Check sheet for the modelled part. Datum: model origin and axes. Units: mm. A direction names the side the tool comes from. Round coordinates to 2 decimals unless told otherwise and drop trailing zeros. Order: outer loops, then holes, each group sorted by start corner. A loop starts at its lowest first (then second) coordinate and runs counter-clockwise, first axis right, second up. Notation, with made-up numbers: M 43.25,8.5 L 54.25,8.5 A6 cw 54.25,13.5 Z; hole C -17,0 d3. An arc over 180 degrees is marked long. One line per item, written item: value. Start each with the question number.
(1) Cross-section at B-B, the plane z = 0. Enter the section's corners in (x, y) (3 decimals), and give its area (3 significant figures).
(2) Cross-section at C-C, the plane y = 3.25. Enter the section's corners in (x, z), and give its area (3 significant figures).
(3) Access from +Z, -Z, +X, -X, +Y, -Y to the whole of each face (thin tool, end or side, straight path). Record for faces 4 (the face through (4, 8, -5)), 5 (the face through (0, 10, -9.975)).
(4) Cross-section at A-A, the plane x = 0. Enter the section's corners in (y, z) (3 decimals).
(5) Depth check by flat-ended pin: pin 1 Ø4 at (x, y) = (-5, 4) entering from -Z; pin 2 Ø3 at (x, y) = (-0.5, 7) entering from +Z (3 decimals); pin 3 Ø4 at (x, y) = (-3, 5.5) entering from -Z. Enter the tip coordinate at first touch or a pass-through.
(6) Thickness scan on L1, parallel to X at y = 5, z = 0; L2, parallel to Y at x = -1.5, z = 6.25; L3, parallel to X at y = 10.25, z = 2.75 (3 decimals). Record the ranges inside material, lowest first.
(7) Release check for a two-part mould opening along X. For faces 1 (the face through (-1.802, 4.056, -5.723)), 2 (the face through (0, 10.5, 0)), 3 (the face through (0, 10, 9.975)) record: released by +X, released by -X, zero draft, split by the parting line, or undercut.
(8) Cross-section at D-D, the plane x = -8.5. Enter the section's corners in (y, z) (3 decimals), and give its area (4 significant figures).
from build123d import *

# Parameters (mm, degrees)
CROQUIS1_W              = 6
CROQUIS1_H              = 8
CROQUIS2_W              = 19.95
CROQUIS2_H              = 19.95
SALIENTE_EXTRUIR1_DEPTH = 5
SKETCH6_R               = 4
CUT_EXTRUDE1_DEPTH      = 10.5


with BuildPart() as part:
    # Croquis1 → Revolución1 (revolve)
    with BuildSketch(Plane(origin=(0, 0, 0), x_dir=(0, 0, -1), z_dir=(1, 0, 0)), mode=Mode.PRIVATE) as revoluci_n1_sk:
        with Locations((-3, 4)):
            Rectangle(CROQUIS1_W, CROQUIS1_H)
    revolve(revoluci_n1_sk.sketch.rotate(Axis((0, 0, 0), (0, 1, 0)), 180), axis=Axis((0, 0, 0), (0, 1, 0)))

    # Croquis2 → Saliente-Extruir1 (add)
    with BuildSketch(Plane(origin=(0, 8, 0), x_dir=(1, 0, 0), z_dir=(0, 1, 0))):
        Rectangle(CROQUIS2_W, CROQUIS2_H)
    extrude(amount=SALIENTE_EXTRUIR1_DEPTH)

    # Sketch6 → Cut-Extrude1 (cut)
    with BuildSketch(Plane.XZ):
        with Locations(Location((0, 0, 0), (0, 0, 270))):
            Circle(SKETCH6_R)
    extrude(amount=-CUT_EXTRUDE1_DEPTH, mode=Mode.SUBTRACT)


solid = part.part
Values found:
1. outline: M -9.975,8 L -6,8 L -6,0 L -4,0 L -4,10.5 L 4,10.5 L 4,0 L 6,0 L 6,8 L 9.975,8 L 9.975,13 L -9.975,13 Z
1. area: 112 mm^2
2. outline: C 0,0 d12; hole C 0,0 d8
2. area: 62.8 mm^2
3. face 4: -Y
3. face 5: -Z, +X, -X, +Y, -Y
4. outline: M 0,-6 L 8,-6 L 8,-9.975 L 13,-9.975 L 13,9.975 L 8,9.975 L 8,6 L 0,6 L 0,4 L 10.5,4 L 10.5,-4 L 0,-4 Z
5. pin 1: z = -5.2
5. pin 2: z = 9.975
5. pin 3: z = -5.92
6. L1: -6 to -4, 4 to 6
6. L2: 8 to 13
6. L3: -9.975 to -2.905, 2.905 to 9.975
7. face 1: split by the parting line
7. face 2: undercut
7. face 3: zero draft
8. outline: M 8,-9.975 L 13,-9.975 L 13,9.975 L 8,9.975 Z
8. area: 99.75 mm^2
